Autodesk Inventor part; units mm, degrees
ref_plane "YZ Plane" through (0, 0, 0) normal (1, 0, 0) x (0, 1, 0)
ref_plane "XZ Plane" through (0, 0, 0) normal (0, 1, 0) x (-1, 0, 0)
ref_plane "XY Plane" through (0, 0, 0) normal (0, 0, 1) x (1, 0, 0)
sketch "Sketch1" plane through (0, 0, 0) normal (0, 0, 1) x (1, 0, 0)
  line L0 (-92.7646, -8.503) -> (-89.7646, -8.503)
  line L1 (-89.7646, -8.503) -> (-89.7646, -11.753)
  line L2 (-89.7646, -11.753) -> (-92.7646, -11.753)
  line L3 (-92.7646, -11.753) -> (-92.7646, -8.503)
  line L4 (-92.7646, -21.6527) -> (-89.7646, -21.6527)
  line L5 (-89.7646, -21.6527) -> (-89.7646, -21.7527)
  line L6 (-89.7646, -21.7527) -> (-92.7646, -21.7527)
  line L7 (-92.7646, -21.7527) -> (-92.7646, -21.6527)
  line L8 (-43.5121, 19.6165) -> (76.4879, 19.6165)
  line L9 (76.4879, 19.6165) -> (76.4879, 99.6165)
  line L10 (76.4879, 99.6165) -> (-43.5121, 99.6165)
  line L11 (-43.5121, 99.6165) -> (-43.5121, 19.6165)
  line L12 (16.4879, 99.6165) -> (16.4879, 19.6165) construction
  line L13 (-43.5121, 59.6165) -> (76.4879, 59.6165) construction
  line L14 (3.9879, 63.1165) -> (7.2379, 63.1165)
  line L15 (7.2379, 63.1165) -> (7.2379, 56.1165)
  line L16 (7.2379, 56.1165) -> (3.9879, 56.1165)
  line L17 (3.9879, 56.1165) -> (3.9879, 63.1165)
  line L18 (3.9879, 59.6165) -> (7.2379, 59.6165) construction
  line L19 (28.9879, 63.1165) -> (25.7379, 63.1165)
  line L20 (25.7379, 63.1165) -> (25.7379, 56.1165)
  line L21 (25.7379, 56.1165) -> (28.9879, 56.1165)
  line L22 (28.9879, 56.1165) -> (28.9879, 63.1165)
  line L23 (28.9879, 59.6165) -> (25.7379, 59.6165) construction
  circle A0 centre (-1.5121, 74.6165) radius 5
  circle A1 centre (34.4879, 74.6165) radius 5
  circle A2 centre (-3.5121, 37.1165) radius 2.5
  circle A3 centre (6.4879, 37.1165) radius 2.5
  circle A4 centre (16.4879, 37.1165) radius 2.5
  circle A5 centre (26.4879, 37.1165) radius 2.5
  circle A6 centre (36.4879, 37.1165) radius 2.5
  circle A7 centre (-3.5121, 44.1165) radius 2.5
  line L24 (-6.0121, 37.1165) -> (-1.0121, 37.1165) construction
  circle A8 centre (-3.5121, 30.1165) radius 2.5
  line L25 (6.4879, 39.6165) -> (6.4879, 34.6165) construction
  circle A9 centre (36.4879, 44.1165) radius 2.5
  circle A10 centre (36.4879, 30.1165) radius 2.5
  circle A11 centre (16.4879, 30.1165) radius 2.5
  line L26 (-43.5121, 99.6165) -> (-53.5121, 99.6165)
  line L27 (-53.5121, 99.6165) -> (-53.5121, 19.6165)
  line L28 (-53.5121, 19.6165) -> (-43.5121, 19.6165)
  line L29 (-43.5121, 19.6165) -> (-43.5121, 99.6165)
  arc A12 (16.4879, 99.6165) -> (-34.1013, 83.0147) centre (13.3048, 23.9368) ccw
  arc A13 (-34.1013, 36.2182) -> (16.4879, 19.6165) centre (13.3048, 95.2961) ccw
  arc A14 (-34.1013, 83.0147) -> (-34.1013, 36.2182) centre (-15.3258, 59.6165) ccw
  arc A15 (67.0771, 83.0147) -> (16.4879, 99.6165) centre (19.6709, 23.9368) ccw
  arc A16 (16.4879, 19.6165) -> (67.0771, 36.2182) centre (19.6709, 95.2961) ccw
  arc A17 (67.0771, 36.2182) -> (67.0771, 83.0147) centre (48.3015, 59.6165) ccw
  line L30 (10.086, 48.1846) -> (0.2957, 56.3433)
  line L31 (3.4966, 65.1844) -> (16.4879, 65.1844)
  arc A18 (3.4966, 65.1844) -> (0.2957, 56.3433) centre (3.4966, 60.1844) ccw
  line L32 (22.8898, 48.1846) -> (32.6801, 56.3433)
  line L33 (29.4791, 65.1844) -> (16.4879, 65.1844)
  arc A19 (32.6801, 56.3433) -> (29.4791, 65.1844) centre (29.4791, 60.1844) ccw
  arc A20 (10.086, 48.1846) -> (22.8898, 48.1846) centre (16.4879, 55.8667) ccw
  point P0 (0, 0)
  point P1 (16.4879, 42.8496)
  dimension "d3" = 3
  dimension "mat" = 3.25
  dimension "d5" = 3
  dimension "kerf" = 0.1
  dimension "d42" = 120
  dimension "d43" = 80
  dimension "d44" = 3.25
  dimension "d45" = 7
  dimension "d47" = 9.25
  dimension "d50" = 10
  dimension "d51" = 13
  dimension "d54" = 20
  dimension "d55" = 5
  dimension "d58" = 10
  dimension "d63" = 15
  dimension "d64" = 5
  dimension "d65" = 7
  dimension "d69" = 10
  dimension "d70" = 30
  dimension "d73" = 5
  dimension "d74" = 10
extrude "Extrusion11" add sketch "Sketch1" along normal blind 3.25 contours L14 L15 L16 L17 | L22 L21 L20 L19 | L30 A18 L31 L33 A19 L32 A20
equation "\"d44\" = mat"
equation "\"d77\" = mat"
properties part number "body-back"
For this review, take the finished solid that the model builds, in its own axes (mm). Coordinates: 2 decimals unless noted, no trailing zeros. Write each loop counter-clockwise with the first axis right and the second up, starting at its lowest first coordinate (ties: lowest second). Pieces come first, ordered by that corner, then holes. Notation, with made-up numbers: (65, 77.25) - (113, 77.25) arc R30 ccw to (113, 116.25) - close; hole circle Ø9 at (-32, -39). An arc over 180 degrees is marked (long way). Answer in a Markdown table with one row per item. Add a question column.
Q1. We need section C-C, the plane y = 55.75. State the section outline as (x, z) points, and give its area (3 significant figures).
Q2. For probe 1 along X at (y, z) = (61.75, 2.35); probe 2 along X at (y, z) = (59.25, 1.2); probe 3 along Y at (x, z) = (22, 1.65), list the stretches that pass through material, from the lowest coordinate up.
Q3. We need section B-B, the plane x = 7. State the section outline as (y, z) points.
Q4. We need section A-A, the plane z = 1.2. State the section outline as (x, y) points, and give its area (3 significant figures).
Q5. For P1, Ø1.5, axis at y = 54.5, z = 2, coming from the +X side; P2, Ø10, axis at x = 7, y = 55.5, coming from the -Z side, all flat-tipped, find the tip position at first contact; note any pin that passes through.
Answer list:
| question | item | result |
|---|---|---|
| 1 | outline | (1.01, 0) - (31.97, 0) - (31.97, 3.25) - (1.01, 3.25) - close |
| 1 | area | 101 mm2 |
| 2 | probe 1 | x = -1.25 to 34.23 |
| 2 | probe 2 | x = -1.42 to 34.39 |
| 2 | probe 3 | y = 47.52 to 65.18 |
| 3 | outline | (50.76, 0) - (65.18, 0) - (65.18, 3.25) - (50.76, 3.25) - close |
| 4 | outline | (0.3, 56.34) - (10.09, 48.18) arc R10 ccw to (22.89, 48.18) - (32.68, 56.34) arc R5 ccw to (29.48, 65.18) - (3.5, 65.18) arc R5 ccw to start |
| 4 | area | 508 mm2 |
| 5 | P1 | stops at x = 31.37 |
| 5 | P2 | stops at z = 0 |
